from build123d import *

# Parameters (mm, degrees)
BOSS_EXTRUDE1_DEPTH = 5
SKETCH4_R           = 0.85
CUT_EXTRUDE3_DEPTH  = 21.432816742
SKETCH5_W           = 4
SKETCH5_H           = 2.5
CUT_EXTRUDE4_DEPTH  = 13
FILLET4_R           = 1
CUT_EXTRUDE5_DEPTH  = 21.432816742
FILLET6_R           = 1
CUT_EXTRUDE6_START  = -8.5
CUT_EXTRUDE6_DEPTH  = 7.974174509
SKETCH11_W          = 2.5
SKETCH11_H          = 5
CUT_EXTRUDE8_DEPTH  = 4
SKETCH12_R          = 0.6
CUT_EXTRUDE9_DEPTH  = 5
SKETCH9_R           = 0.25
CUT_EXTRUDE10_DEPTH = 8.5
FILLET7_R           = 1


# Read off the part's stored shape, not the designer's step: Cut-Extrude6
with BuildPart() as part:
    # Sketch1 → Boss-Extrude1 (new body)
    with BuildSketch(Plane.XY):
        Polygon((0, 0), (13.5, 0), (13.5, -14.5), (8, -14.5), (8, -5), (0, -5), align=None)
    extrude(amount=BOSS_EXTRUDE1_DEPTH)

    # Sketch4 → Cut-Extrude3 (cut, through all)
    with BuildSketch(Plane.XY.offset(5)):
        with Locations((1.75, -2.5)):
            Circle(SKETCH4_R)
    extrude(amount=-CUT_EXTRUDE3_DEPTH, mode=Mode.SUBTRACT)

    # Sketch5 → Cut-Extrude4 (cut)
    with BuildSketch(Plane(origin=(0, 0, 0), x_dir=(1, 0, 0), z_dir=(0, 1, 0))):
        with Locations((2, -2.5)):
            Rectangle(SKETCH5_W, SKETCH5_H)
    extrude(amount=-CUT_EXTRUDE4_DEPTH, mode=Mode.SUBTRACT)

    # Fillet4
    fillet4_edges = [part.edges().sort_by_distance(p)[0] for p in [
        (0, 0, 4.375),
        (0, -5, 4.375),
        (0, 0, 0.625),
        (0, -5, 0.625),
    ]]
    fillet(fillet4_edges, radius=FILLET4_R)

    # Sketch6 → Cut-Extrude5 (cut, through all)
    with BuildSketch(Plane.XY.offset(5)):
        Polygon((13.5, -13.588182425), (12.5, -12.588182425), (13.5, -11.588182425), align=None)
    extrude(amount=-CUT_EXTRUDE5_DEPTH, mode=Mode.SUBTRACT)

    # Fillet6
    fillet6_edges = [part.edges().sort_by_distance(p)[0] for p in [
        (12.5, -12.588182425, 2.5),
        (13.5, -13.588182425, 2.5),
        (13.5, -11.588182425, 2.5),
        (8, -5, 2.5),
        (8, -14.5, 2.5),
        (13.5, 0, 2.5),
    ]]
    fillet(fillet6_edges, radius=FILLET6_R - 0.0001)  # a hair under: the kernel refuses the full size

    # Cut-Extrude6 outline → Cut-Extrude6 (cut)
    with BuildSketch(Plane.XZ.offset(14.5).offset(CUT_EXTRUDE6_START)):
        with BuildLine():
            Line((7.999994957, 5.000049402), (7.999994964, 0.302944212))
            ThreePointArc((7.999994964, 0.302944212), (8.119562434, 2.651496807), (7.999994957, 5.000049402))
        make_face()
    extrude(amount=CUT_EXTRUDE6_DEPTH, mode=Mode.SUBTRACT)

    # Sketch11 → Cut-Extrude8 (cut, along a direction that is not the sketch's normal)
    with BuildSketch(Plane.ZY.offset(-4)):
        with Locations((2.5, -2.5)):
            Rectangle(SKETCH11_W, SKETCH11_H)
    extrude(amount=-CUT_EXTRUDE8_DEPTH, dir=(-0.894528038262942, 0.4470118440952684, 0), mode=Mode.SUBTRACT)

    # Sketch12 → Cut-Extrude9 (cut, along a direction that is not the sketch's normal)
    with BuildSketch(Plane.ZY.offset(-8)):
        with Locations((3.671694189, -8.375443102)):
            Circle(SKETCH12_R)
        with Locations((3.671694189, -10.194652501)):
            Circle(SKETCH12_R)
        with Locations((3.671694189, -12.168032187)):
            Circle(SKETCH12_R)
        with Locations((2.5, -6)):
            Circle(SKETCH12_R)
    extrude(amount=-CUT_EXTRUDE9_DEPTH, dir=(-0.894528038262942, 0.4470118440952684, 0), mode=Mode.SUBTRACT)

    # Sketch9 → Cut-Extrude10 (cut)
    with BuildSketch(Plane.XZ.offset(14.5)):
        with Locations((8.119066185, 2.5)):
            Circle(SKETCH9_R)
    extrude(amount=-CUT_EXTRUDE10_DEPTH, mode=Mode.SUBTRACT)

    # Fillet7
    fillet7_edges = [part.edges().sort_by_distance(p)[0] for p in [
        (5.789056077, -0.894023688, 1.25),
        (5.789056077, -0.894023688, 3.75),
        (7.578112153, -3.486020884, 3.75),
        (7.578112153, -3.486020884, 1.25),
    ]]
    fillet(fillet7_edges, radius=FILLET7_R)


solid = part.part
Design review of the part built by this model. Coordinates are the model's own, in mm. A direction names the side the tool comes from. Round coordinates to 2 decimals unless told otherwise and drop trailing zeros. Loops run counter-clockwise (first coordinate to the right, second up) from the corner with the lowest first, then second, coordinate; pieces in that order, holes last. Notation, with made-up numbers: (-22, -23.5) -> (1, -23.5) arc R34 cw to (1, 6.5) -> close; hole circle Ø7 at (34.5, 17.5). An arc over 180 degrees is marked (long way). Use one line per item in the form item = value. Start each with the question number.
Q1. For pin 1 Ø1.5 at (x, z) = (3.5, 0.5) entering from -Y; pin 2 Ø0.6 at (y, z) = (-9.5, 0.5) entering from -X; pin 3 Ø1.5 at (x, y) = (2, -2.5) entering from -Z; pin 4 Ø1.3 at (y, z) = (-10.5, 3.5) entering from -X, all flat-tipped, find the tip position at first contact; note any pin that passes through.
Q2. We need section A-A on y = -3.75. Give the boundary of the cut face in (x, z).
Q3. Draft analysis for pull direction Z (two halves, no side actions). For faces 6 (the face through (12.473, -12.4, 3.7)), 7 (the face through (8.3, -5.5, 5)), 8 (the face through (4, -5, 4)), state which applies: +Z half, -Z half, draft (parallel to the pull), parting line (faces both ways), or undercut.
Q4. Machinability: for faces 1 (the face through (2.535, -2.826, 4.384)), 2 (the face through (4, -5, 1)), 3 (the face through (12.473, -10.6, 3.7)), 4 (the face through (8.056, -9.931, 4.361)), 5 (the face through (12.914, -12.599, 2.465)), which of the approach directions +Z, -Z, +X, -X, +Y, -Y give a long, thin tool a straight path to every point of the face, cutting with its end or side? Answer none if there is none.
Q5. Wall thickness on line 1 along Y through (x, z) = (1.75, 0.95); line 2 along Z through (x, y) = (5.25, -2); line 3 along Y through (x, z) = (6.25, 3.9): over which ranges is each line inside the solid? List them lowest first. Write a range as [from, to].
Calculated:
q1.pin_1 = -5
q1.pin_2 = 8
q1.pin_3 = 0
q1.pin_4 = 8.07
q2.outline = (0, 0) -> (13.5, 0) -> (13.5, 5) -> (0, 5) -> (0, 3.75) -> (6.58, 3.75) arc R1 cw to (7.58, 2.75) -> (7.58, 2.25) arc R1 cw to (6.58, 1.25) -> (0, 1.25) -> close
q3.face_6 = undercut
q3.face_7 = +Z half
q3.face_8 = draft
q4.face_1 = +Z, -Z
q4.face_2 = +Z, -Z, -X, -Y
q4.face_3 = none
q4.face_4 = -X, -Y
q4.face_5 = +Z, -Z, +X
q5.line_1 = [-5, -3.35], [-1.65, 0]
q5.line_2 = [0, 1.25], [3.75, 5]
q5.line_3 = [-5, 0]
